Answer from the drawing. Dimensions are ordinates in mm from the lowest x, y and z of the part. Round coordinates to 2 decimals unless told otherwise and drop trailing zeros. Loops run counter-clockwise (first coordinate to the right, second up) from the corner with the lowest first, then second, coordinate; pieces in that order, holes last.
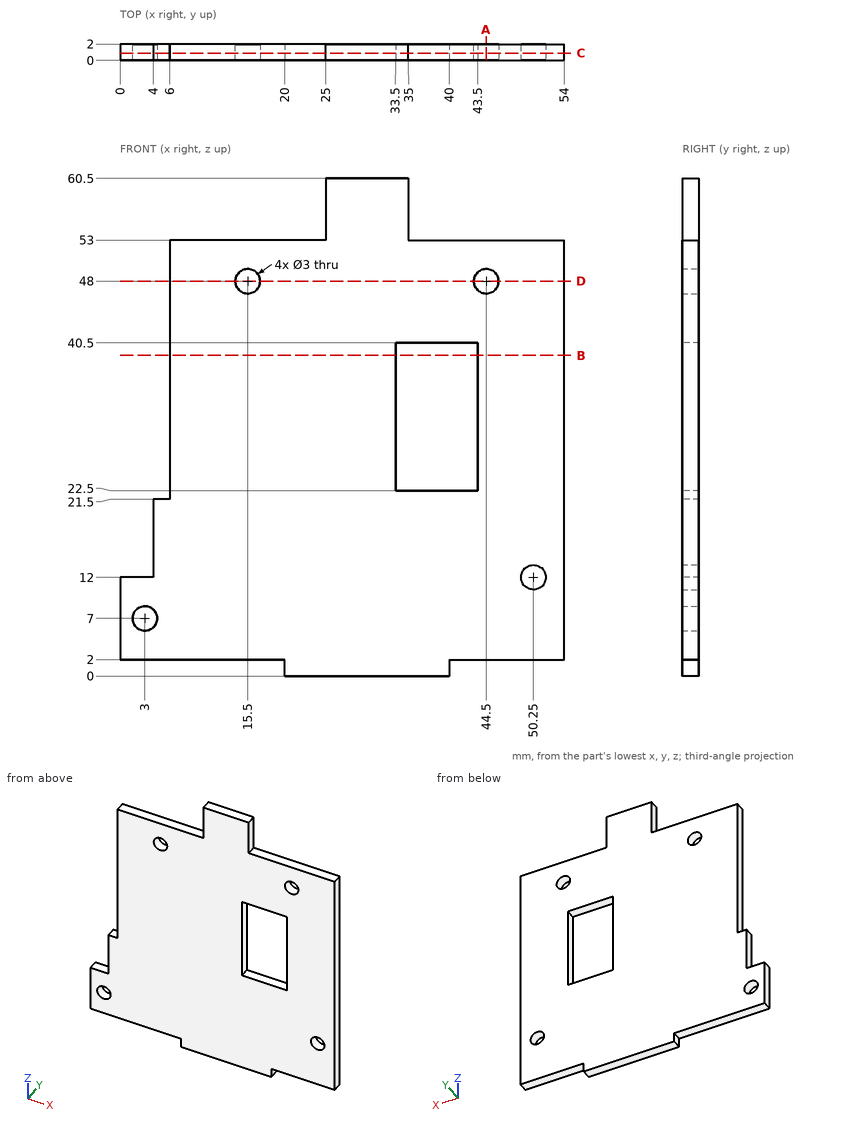
1. Find section A-A (x = 44.5). Write down the section's boundary in (y, z), then the cut area to 3 significant figures.
Answer key:
outline: (0, 2) - (2, 2) - (2, 46.5) - (0, 46.5) - close; (0, 49.5) - (2, 49.5) - (2, 53) - (0, 53) - close
area: 96.0 mm2
2. Find section C-C (y = 0.9). Write down the section's boundary in (x, z).
Answer key:
outline: (0, 2) - (20, 2) - (20, 0) - (40, 0) - (40, 2) - (54, 2) - (54, 53) - (35, 53) - (35, 60.5) - (25, 60.5) - (25, 53) - (6, 53) - (6, 21.5) - (4, 21.5) - (4, 12) - (0, 12) - close; hole circle Ø3 at (3, 7); hole circle Ø3 at (15.5, 48); hole (33.5, 22.5) - (43.5, 22.5) - (43.5, 40.5) - (33.5, 40.5) - close; hole circle Ø3 at (44.5, 48); hole circle Ø3 at (50.25, 12)
3. Find section D-D (z = 48). Write down the section's boundary in (x, y), then the cut area to 3 significant figures.
Answer key:
outline: (6, 0) - (14, 0) - (14, 2) - (6, 2) - close; (17, 0) - (43, 0) - (43, 2) - (17, 2) - close; (46, 0) - (54, 0) - (54, 2) - (46, 2) - close
area: 84.0 mm2
4. Consider probe 1 along X at (y, z) = (1.2, 48); probe 2 along Z at (x, y) = (44.5, 0.4); probe 3 along X at (y, z) = (1.6, 25). Determine where each line is inside the solid, lowest interval first.
Answer key:
probe 1: x = 6 to 14, 17 to 43, 46 to 54
probe 2: z = 2 to 46.5, 49.5 to 53
probe 3: x = 6 to 33.5, 43.5 to 54
5. Find section B-B (z = 39). Write down the section's boundary in (x, y).
Answer key:
outline: (6, 0) - (33.5, 0) - (33.5, 2) - (6, 2) - close; (43.5, 0) - (54, 0) - (54, 2) - (43.5, 2) - close
6. Given pin 1 (0.6 mm diameter, centred on x = 43, y = 1, fed in from +Z); pin 2 (0.6 mm diameter, centred on y = 1, z = 32.5, fed in from -X); pin 3 (0.6 mm diameter, centred on y = 1.5, z = 1.5, fed in from +X), each flat-ended and moving along its own axis, determine where each tip first touches the part or whether it passes through.
Answer key:
pin 1: stops at z = 53
pin 2: stops at x = 6
pin 3: stops at x = 40
